Verification items for the finished model (mm, model axes). A direction names the side the tool comes from. Round coordinates to 2 decimals unless told otherwise and drop trailing zeros. Write each loop counter-clockwise with the first axis right and the second up, starting at its lowest first coordinate (ties: lowest second). Pieces come first, ordered by that corner, then holes. Notation, with made-up numbers: (-27, 61) -> (9, 61) arc R6 cw to (9, 68) -> close; hole circle Ø8 at (61, 46). An arc over 180 degrees is marked (long way). Answer as a JSON object with one key per item and string values. Group by question number.
(1) Gauge pin test, flat ends, axial feed: pin 1 Ø2.5 at (x, z) = (-5, 3.5) entering from +Y; pin 2 Ø2.5 at (y, z) = (-16, 1.5) entering from -X; pin 3 Ø1.5 at (y, z) = (17.5, 3) entering from +X; pin 4 Ø5 at (x, y) = (0, -15) entering from -Z. Record the tip position at first contact, or that the pin passes through.
(2) Scan lines: L1, parallel to Y at x = 6.5, z = 2.1; L2, parallel to X at y = 7, z = 4.5. Record each from-to range of solid material in increasing order. Write a range as from..to.
(3) Set-up check for faces 1 (the face through (5, 7.5, 3)), 2 (the face through (-5, 7.5, 3)), 3 (the face through (-5, 12.5, 2)): record each of +Z, -Z, +X, -X, +Y, -Y from which the full face is reachable in a straight line by a thin tool's end or side.
(4) Sectioned sample at A-A on x = -4.5. Record the cut outline in (y, z).
(5) Draft check along Y on faces 4 (the face through (7.5, 10, 2)), 5 (the face through (0, 20, 2)), 6 (the face through (2.5, 5, 3)), 7 (the face through (-5, -7.5, 3)). Enter one of: released by +Y, released by -Y, zero draft, split by the parting line, or undercut.
(6) Sectioned sample at B-B on z = 1.25. Record the cut outline in (x, y).
(7) Sectioned sample at C-C on y = -5. Record the cut outline in (x, z).
```python
from build123d import *

# Parameters (mm, degrees)
ESQUISSE6_W               = 15
ESQUISSE6_H               = 40
BOSS_EXTRU_3_DEPTH        = 5
ESQUISSE7_W               = 5
ESQUISSE7_H               = 7.5
ENL_V_MAT_EXTRU_4_DEPTH   = 5
SYM_TRIE4_COPY_1_SKETCH_W = 5
SYM_TRIE4_COPY_1_SKETCH_H = 7.5
SYM_TRIE4_COPY_1_DEPTH    = 5
ESQUISSE9_W               = 5
ESQUISSE9_H               = 5
ENL_V_MAT_EXTRU_6_DEPTH   = 5
SYM_TRIE6_COPY_1_SKETCH_W = 5
SYM_TRIE6_COPY_1_SKETCH_H = 5
SYM_TRIE6_COPY_1_DEPTH    = 5


with BuildPart() as part:
    # Esquisse6 → Boss.-Extru.3 (new body)
    with BuildSketch(Plane.XY):
        Rectangle(ESQUISSE6_W, ESQUISSE6_H)
    extrude(amount=BOSS_EXTRU_3_DEPTH)

    # Esquisse7 → Enlèv. mat.-Extru.4 (cut)
    with BuildSketch(Plane.XY):
        with Locations((-5, 16.25)):
            Rectangle(ESQUISSE7_W, ESQUISSE7_H)
    enl_v_mat_extru_4 = extrude(amount=ENL_V_MAT_EXTRU_4_DEPTH, mode=Mode.SUBTRACT)

    # Symétrie3: Enlèv. mat.-Extru.4 across plane
    add(enl_v_mat_extru_4.mirror(Plane.ZX), mode=Mode.SUBTRACT)

    # Symétrie4: Enlèv. mat.-Extru.4 across plane
    add(enl_v_mat_extru_4.mirror(Plane(origin=(0, 0, 0), x_dir=(0, 0, 1), z_dir=(1, 0, 0))), mode=Mode.SUBTRACT)

    # Symétrie4 copy 1 sketch → Symétrie4 copy 1 (cut)
    with BuildSketch(Plane(origin=(0, 0, 0), x_dir=(-1, 0, 0), z_dir=(0, 0, 1))):
        with Locations((-5, 16.25)):
            Rectangle(SYM_TRIE4_COPY_1_SKETCH_W, SYM_TRIE4_COPY_1_SKETCH_H)
    extrude(amount=SYM_TRIE4_COPY_1_DEPTH, mode=Mode.SUBTRACT)

    # Esquisse9 → Enlèv. mat.-Extru.6 (cut)
    with BuildSketch(Plane.XY.offset(5)):
        with Locations((-5, 5)):
            Rectangle(ESQUISSE9_W, ESQUISSE9_H)
    enl_v_mat_extru_6 = extrude(amount=-ENL_V_MAT_EXTRU_6_DEPTH, mode=Mode.SUBTRACT)

    # Symétrie5: Enlèv. mat.-Extru.6 across plane
    add(enl_v_mat_extru_6.mirror(Plane.ZX), mode=Mode.SUBTRACT)

    # Symétrie6: Enlèv. mat.-Extru.6 across plane
    add(enl_v_mat_extru_6.mirror(Plane(origin=(0, 0, 0), x_dir=(0, 0, 1), z_dir=(1, 0, 0))), mode=Mode.SUBTRACT)

    # Symétrie6 copy 1 sketch → Symétrie6 copy 1 (cut)
    with BuildSketch(Plane(origin=(0, 0, 5), x_dir=(-1, 0, 0), z_dir=(0, 0, 1))):
        with Locations((-5, 5)):
            Rectangle(SYM_TRIE6_COPY_1_SKETCH_W, SYM_TRIE6_COPY_1_SKETCH_H)
    extrude(amount=-SYM_TRIE6_COPY_1_DEPTH, mode=Mode.SUBTRACT)


solid = part.part
```
Computed values:
{
 "1": {"pin 1": "y = 12.5", "pin 2": "x = -2.5", "pin 3": "x = 2.5", "pin 4": "z = 0"},
 "2": {"L1": "-12.5..-7.5, -2.5..2.5, 7.5..12.5", "L2": "-2.5..2.5"},
 "3": {"face 1": "+Z, -Z, +X", "face 2": "+Z, -Z, -X", "face 3": "+Z, -Z, -X, +Y"},
 "4": {"outline": "(-12.5, 0) -> (-7.5, 0) -> (-7.5, 5) -> (-12.5, 5) -> close; (-2.5, 0) -> (2.5, 0) -> (2.5, 5) -> (-2.5, 5) -> close; (7.5, 0) -> (12.5, 0) -> (12.5, 5) -> (7.5, 5) -> close"},
 "5": {"face 4": "zero draft", "face 5": "released by +Y", "face 6": "undercut", "face 7": "undercut"},
 "6": {"outline": "(-7.5, -12.5) -> (-2.5, -12.5) -> (-2.5, -20) -> (2.5, -20) -> (2.5, -12.5) -> (7.5, -12.5) -> (7.5, -7.5) -> (2.5, -7.5) -> (2.5, -2.5) -> (7.5, -2.5) -> (7.5, 2.5) -> (2.5, 2.5) -> (2.5, 7.5) -> (7.5, 7.5) -> (7.5, 12.5) -> (2.5, 12.5) -> (2.5, 20) -> (-2.5, 20) -> (-2.5, 12.5) -> (-7.5, 12.5) -> (-7.5, 7.5) -> (-2.5, 7.5) -> (-2.5, 2.5) -> (-7.5, 2.5) -> (-7.5, -2.5) -> (-2.5, -2.5) -> (-2.5, -7.5) -> (-7.5, -7.5) -> close"},
 "7": {"outline": "(-2.5, 0) -> (2.5, 0) -> (2.5, 5) -> (-2.5, 5) -> close"}
}
